```python
from build123d import *

# Parameters (mm, degrees)
F0_W     = 96.798718
F0_H     = 133.88981
F1_DEPTH = 19.05
F2_W     = 96.798718
F2_H     = 25.068198
F3_DEPTH = 38.1
F4_W     = 25.4
F4_H     = 25.068198
F5_DEPTH = 19.05
F6_R     = 24.355742
F7_DEPTH = 19.051
F8_R     = 25.4
F9_R     = 25.4


with BuildPart() as f1:
    # F0 (on Front) → F1 (new body)
    with BuildSketch(Plane.XZ):
        Rectangle(F0_W, F0_H)
    extrude(amount=F1_DEPTH)

    # F2 (on face) → F3 (join)
    with BuildSketch(Plane.XZ.offset(19.05)):
        with Locations((0, -54.410806)):
            Rectangle(F2_W, F2_H)
    extrude(amount=F3_DEPTH)

    # F4 (on face) → F5 (cut)
    with BuildSketch(Plane.XZ.offset(57.15)):
        with Locations((35.699359, -54.410806)):
            Rectangle(F4_W, F4_H)
    extrude(amount=-F5_DEPTH, mode=Mode.SUBTRACT)

    # F6 (on face) → F7 (cut, through all)
    with BuildSketch(Plane.XZ.offset(19.05)):
        with Locations((0, 30.258423)):
            Circle(F6_R)
    extrude(amount=-F7_DEPTH, mode=Mode.SUBTRACT)

    # F8
    f8_edges = [f1.edges().sort_by_distance(p)[0] for p in [
        (-48.399359, -9.525, 66.944905),
    ]]
    fillet(f8_edges, radius=F8_R)

    # F9
    f9_edges = [f1.edges().sort_by_distance(p)[0] for p in [
        (48.399359, -9.525, 66.944905),
    ]]
    fillet(f9_edges, radius=F9_R)


solid = f1.part
```
Work out the finished part from the listing and answer in its coordinate system (mm). A direction names the side the tool comes from. Give positions to 0.01 mm unless a question says otherwise; leave off trailing zeros. Loops run counter-clockwise (first coordinate to the right, second up) from the corner with the lowest first, then second, coordinate; pieces in that order, holes last. Notation, with made-up numbers: (24.5, 30.25) -> (47.5, 30.25) arc R11 cw to (47.5, 43.25) -> close; hole circle Ø8 at (8, 23). An arc over 180 degrees is marked (long way). Put each result on its own line as item: value. Start each with the question number.
Item 1: Each of these flat-tipped pins is pushed along its axis until it touches: P1, Ø12.5, axis at x = 33.5, z = -59, coming from the -Y side; P2, Ø6, axis at x = 15.5, y = -23.5, coming from the +Z side; P3, Ø5.5, axis at y = -43.5, z = -49.5, coming from the +X side. Where does it stop, or does it pass through?
Item 2: Which of the six approach directions +Z, -Z, +X, -X, +Y, -Y give full straight-line access (tool end or side, diameter ignored) to faces 5 (the face through (-13, -57.15, -54)), 6 (the face through (22.999, -48, -55)), 7 (the face through (-1, -19.05, 1))?
Item 3: Find the intervals of material crossed by L1, parallel to Z at x = 0, y = -6; L2, parallel to Y at x = 1.5, z = -10; L3, parallel to Y at x = 41, z = -61, in increasing order. Write a range as [from, to].
Item 4: The part is cut by section C-C (y = -10.5). Give the vertices of the cut face in (x, z), then the cut area to 3 significant figures.
Item 5: The part is cut by section A-A (x = 0). Give the vertices of the cut face in (y, z), then the cut area to 3 significant figures.
Item 6: The part is cut by section D-D (y = -48.5). Give the vertices of the cut face in (x, z), then the cut area to 3 significant figures.
Item 7: The part is cut by section B-B (z = 26). Give the vertices of the cut face in (x, y).
Item 8: The mould has two halves that part along Z. Classify faces 1 (the face through (48.399, -15, -26)), 2 (the face through (-3.171, -9.658, 54.407)), 3 (the face through (-1, -28, -66.945)), 4 (the face through (-1, -38, -41.877)): released by +Z, released by -Z, zero draft, split by the parting line, or undercut.
Answers below:
1. P1: y = -38.1
1. P2: z = -41.88
1. P3: x = 23
2. face 5: +Z, -Z, +X, -X, -Y
2. face 6: +Z, -Z, +X, -Y
2. face 7: +Z, +X, -X, -Y
3. L1: [-66.94, 5.9], [54.61, 66.94]
3. L2: [-19.05, 0]
3. L3: [-38.1, 0]
4. outline: (-48.4, -66.94) -> (48.4, -66.94) -> (48.4, 41.54) arc R25.4 ccw to (23, 66.94) -> (-23, 66.94) arc R25.4 ccw to (-48.4, 41.54) -> close; hole circle Ø48.71 at (0, 30.26)
4. area: 10,800 mm2
5. outline: (-57.15, -66.94) -> (0, -66.94) -> (0, 5.9) -> (-19.05, 5.9) -> (-19.05, -41.88) -> (-57.15, -41.88) -> close; (-19.05, 54.61) -> (0, 54.61) -> (0, 66.94) -> (-19.05, 66.94) -> close
5. area: 2,580 mm2
6. outline: (-48.4, -66.94) -> (23, -66.94) -> (23, -41.88) -> (-48.4, -41.88) -> close
6. area: 1,790 mm2
7. outline: (-48.4, -19.05) -> (-23.98, -19.05) -> (-23.98, 0) -> (-48.4, 0) -> close; (23.98, -19.05) -> (48.4, -19.05) -> (48.4, 0) -> (23.98, 0) -> close
8. face 1: zero draft
8. face 2: undercut
8. face 3: released by -Z
8. face 4: released by +Z
